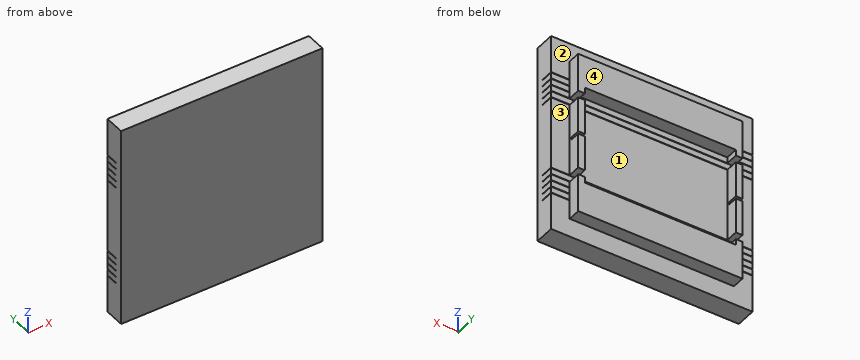
Autodesk Inventor part; units mm, degrees
ref_plane "YZ Plane" through (0, 0, 0) normal (1, 0, 0) x (0, 1, 0)
ref_plane "XZ Plane" through (0, 0, 0) normal (0, 1, 0) x (-1, 0, 0)
ref_plane "XY Plane" through (0, 0, 0) normal (0, 0, 1) x (1, 0, 0)
sketch "Boceto1" plane through (0, 0, 0) normal (0, 1, 0) x (-1, 0, 0)
  line L0 (0, 0) -> (80, 0)
  line L1 (80, 0) -> (80, -80)
  line L2 (80, -80) -> (0, -80)
  line L3 (0, -80) -> (0, 0)
  line L4 (10, -70) -> (70, -70)
  line L5 (70, -70) -> (70, -10)
  line L6 (70, -10) -> (10, -10)
  line L7 (10, -10) -> (10, -70)
  line L8 (0, -12.375) -> (80, -12.375)
  line L9 (0, -14.95) -> (80, -14.95)
  line L10 (0, -17.525) -> (80, -17.525)
  line L11 (80, -20.1) -> (0, -20.1)
  line L12 (0, -22.675) -> (80, -22.675)
  line L13 (0, -12.575) -> (80, -12.575)
  line L14 (0, -15.15) -> (80, -15.15)
  line L15 (0, -17.725) -> (80, -17.725)
  line L16 (80, -20.3) -> (0, -20.3)
  line L17 (0, -22.875) -> (80, -22.875)
  line L18 (0, -25.25) -> (80, -25.25)
  line L19 (0, -25.45) -> (80, -25.45)
  line L20 (10, -40) -> (80, -40)
  line L21 (0, -67.625) -> (80, -67.625)
  line L22 (0, -65.05) -> (80, -65.05)
  line L23 (0, -62.475) -> (80, -62.475)
  line L24 (80, -59.9) -> (0, -59.9)
  line L25 (0, -57.325) -> (80, -57.325)
  line L26 (0, -67.425) -> (80, -67.425)
  line L27 (0, -64.85) -> (80, -64.85)
  line L28 (0, -62.275) -> (80, -62.275)
  line L29 (80, -59.7) -> (0, -59.7)
  line L30 (0, -57.125) -> (80, -57.125)
  line L31 (0, -54.75) -> (80, -54.75)
  line L32 (0, -54.55) -> (80, -54.55)
  line L33 (72.625, -7.375) -> (7.375, -7.375)
  line L34 (7.375, -7.375) -> (7.375, -72.625)
  line L35 (7.375, -72.625) -> (72.625, -72.625)
  line L36 (72.625, -72.625) -> (72.625, -7.375)
  line L37 (7.375, 0) -> (0, 0)
  line L38 (7.375, -80) -> (0, -80)
  point P0 (10, -12.375)
  point P1 (70, -12.375)
  point P2 (10, -14.95)
  point P3 (70, -14.95)
  point P4 (10, -17.525)
  point P5 (70, -17.525)
  point P6 (70, -20.1)
  point P7 (10, -20.1)
  point P8 (10, -22.675)
  point P9 (70, -22.675)
  point P10 (10, -12.575)
  point P11 (70, -12.575)
  point P12 (10, -15.15)
  point P13 (70, -15.15)
  point P14 (10, -17.725)
  point P15 (70, -17.725)
  point P16 (70, -20.3)
  point P17 (10, -20.3)
  point P18 (10, -22.875)
  point P19 (70, -22.875)
  point P20 (10, -25.25)
  point P21 (70, -25.25)
  point P22 (10, -25.45)
  point P23 (70, -25.45)
  point P24 (10, -67.625)
  point P25 (70, -67.625)
  point P26 (10, -65.05)
  point P27 (70, -65.05)
  point P28 (10, -62.475)
  point P29 (70, -62.475)
  point P30 (70, -59.9)
  point P31 (10, -59.9)
  point P32 (10, -57.325)
  point P33 (70, -57.325)
  point P34 (10, -67.425)
  point P35 (70, -67.425)
  point P36 (10, -64.85)
  point P37 (70, -64.85)
  point P38 (10, -62.275)
  point P39 (70, -62.275)
  point P40 (70, -59.7)
  point P41 (10, -59.7)
  point P42 (10, -57.125)
  point P43 (70, -57.125)
  point P44 (10, -54.75)
  point P45 (70, -54.75)
  point P46 (10, -54.55)
  point P47 (70, -54.55)
  point P48 (72.625, -12.375)
  point P49 (7.375, -12.375)
  point P50 (72.625, -54.55)
  point P51 (72.625, -25.45)
  point P52 (70, -25.45)
  point P53 (70, -54.55)
  point P54 (7.375, -25.45)
  point P55 (7.375, -54.55)
  point P56 (10, -54.55)
  point P57 (10, -25.45)
  point P58 (10, -67.625)
  point P59 (7.375, -67.625)
  point P60 (72.625, -67.625)
  point P61 (70, -67.625)
  point P62 (7.375, -14.95)
  point P63 (72.625, -14.95)
  point P64 (72.625, -65.05)
  point P65 (70, -65.05)
  point P66 (10, -65.05)
  point P67 (7.375, -65.05)
  point P68 (70, -67.425)
  point P69 (10, -67.425)
  point P70 (10, -12.575)
  point P71 (70, -12.575)
  point P72 (72.625, -64.85)
  point P73 (7.375, -64.85)
  point P74 (7.375, -15.15)
  point P75 (70, -15.15)
  point P76 (7.375, -62.475)
  point P77 (10, -64.85)
  point P78 (10, -62.475)
  point P79 (72.625, -62.475)
  point P80 (70, -62.475)
  point P81 (70, -64.85)
  point P82 (7.375, -17.525)
  point P83 (10, -15.15)
  point P84 (72.625, -17.525)
  point P85 (72.625, -20.1)
  point P86 (7.375, -20.1)
  point P87 (72.625, -59.9)
  point P88 (70, -59.9)
  point P89 (70, -62.275)
  point P90 (10, -62.275)
  point P91 (10, -59.9)
  point P92 (7.375, -59.9)
  point P93 (10, -17.725)
  point P94 (70, -17.725)
  point P95 (72.625, -57.325)
  point P96 (70, -57.325)
  point P97 (70, -59.7)
  point P98 (10, -59.7)
  point P99 (10, -57.325)
  point P100 (7.375, -57.325)
  point P101 (7.375, -22.675)
  point P102 (10, -20.3)
  point P103 (70, -20.3)
  point P104 (72.625, -22.675)
  dimension "d5" = 10
  dimension "d0" = 80
  dimension "d1" = 80
  dimension "d2" = 60
  dimension "d3" = 60
  dimension "d4" = 10
  dimension "d6" = 2.375
  dimension "d7" = 0.2
  dimension "d8" = 2.375
  dimension "d9" = 0.2
  dimension "d10" = 0.2
  dimension "d11" = 0.2
  dimension "d12" = 0.2
  dimension "d13" = 2.375
  dimension "d14" = 2.375
  dimension "d15" = 2.375
  dimension "d16" = 2.375
  dimension "d17" = 0.2
  dimension "d35" = 5
extrude "Extrusión1" add sketch "Boceto1" along normal blind 5 contours L0 L1 L8 L36 L33 L34 L3 | L8 L34 L13 L3 | L13 L34 L9 L3 | L34 L33 L36 L8 L5 L6 L7 | L8 L7 L13 L34 | L1 L13 L36 L8 | L13 L7 L9 L34 | L8 L5 L13 L7 | L7 L6 L5 L8 | L1 L9 L36 L13 | L36 L13 L5 L8 | L14 L34 L10 L3 | L13 L5 L9 L7 | L36 L9 L5 L13 | L14 L7 L10 L34 | L1 L10 L36 L14 | L15 L34 L11 L3 | L14 L5 L10 L7 | L36 L10 L5 L14 | L15 L7 L11 L34 | L1 L11 L36 L15 | L16 L34 L12 L3 | L15 L5 L11 L7 | L36 L11 L5 L15 | L16 L7 L12 L34 | L1 L12 L36 L16 | L17 L34 L18 L3 | L16 L5 L12 L7 | L36 L12 L5 L16 | L17 L7 L18 L34 | L1 L18 L36 L17 | L19 L34 L32 L3 | L17 L5 L18 L7 | L36 L18 L5 L17 | L19 L7 L32 L34 | L1 L20 L36 L19 | L31 L34 L30 L3 | L19 L5 L20 L7 | L1 L32 L36 L20 | L36 L20 L5 L19 | L31 L7 L30 L34 | L7 L20 L5 L32 | L36 L32 L5 L20 | L25 L34 L29 L3 | L31 L5 L30 L7 | L1 L30 L36 L31 | L25 L7 L29 L34 | L31 L36 L30 L5 | L24 L34 L28 L3 | L25 L5 L29 L7 | L1 L29 L36 L25 | L24 L7 L28 L34 | L25 L36 L29 L5 | L23 L34 L27 L3 | L24 L5 L28 L7 | L1 L28 L36 L24 | L23 L7 L27 L34 | L24 L36 L28 L5 | L22 L34 L26 L3 | L23 L5 L27 L7 | L1 L27 L36 L23 | L26 L34 L21 L3 | L22 L7 L26 L34 | L23 L36 L27 L5 | L21 L34 L35 L36 L1 L2 L3 | L26 L7 L21 L34 | L22 L5 L26 L7 | L1 L26 L36 L22 | L21 L7 L4 L5 L36 L35 L34 | L26 L5 L21 L7 | L22 L36 L26 L5 | L1 L21 L36 L26 | L21 L5 L4 L7 | L26 L36 L21 L5
sketch "Boceto2" plane through (0, 0, 0) normal (0, -1, 0) x (1, 0, 0)
  line L0 (0, -80) -> (-80, -80)
  line L1 (-80, 0) -> (0, 0)
  line L2 (-80, -80) -> (-80, 0)
  line L3 (-80, 0) -> (0, 0)
  line L4 (-80, -65.05) -> (0, -65.05) construction
  line L5 (0, 0) -> (0, -80)
  line L6 (-80, -80) -> (0, -80)
extrude "Extrusión4" add sketch "Boceto2" along normal blind 3
extrude "Extrusión5" add sketch "Boceto1" along normal blind 10 contours L34 L33 L36 L8 L5 L6 L7 | L8 L7 L13 L34 | L13 L7 L9 L34 | L8 L5 L13 L7 | L7 L6 L5 L8 | L36 L13 L5 L8 | L9 L7 L14 L34 | L13 L5 L9 L7 | L36 L9 L5 L13 | L14 L7 L10 L34 | L9 L5 L14 L7 | L36 L14 L5 L9 | L10 L7 L15 L34 | L14 L5 L10 L7 | L36 L10 L5 L14 | L15 L7 L11 L34 | L10 L5 L15 L7 | L36 L15 L5 L10 | L11 L7 L16 L34 | L15 L5 L11 L7 | L36 L11 L5 L15 | L16 L7 L12 L34 | L11 L5 L16 L7 | L36 L16 L5 L11 | L36 L12 L5 L16 | L19 L7 L32 L34 | L36 L20 L5 L19 | L36 L32 L5 L20 | L25 L7 L29 L34 | L29 L7 L24 L34 | L24 L7 L28 L34 | L29 L5 L24 L7 | L25 L36 L29 L5 | L28 L7 L23 L34 | L24 L5 L28 L7 | L29 L36 L24 L5 | L23 L7 L27 L34 | L28 L5 L23 L7 | L24 L36 L28 L5 | L27 L7 L22 L34 | L23 L5 L27 L7 | L28 L36 L23 L5 | L22 L7 L26 L34 | L27 L5 L22 L7 | L23 L36 L27 L5 | L26 L7 L21 L34 | L22 L5 L26 L7 | L27 L36 L22 L5 | L21 L7 L4 L5 L36 L35 L34 | L26 L5 L21 L7 | L22 L36 L26 L5 | L21 L5 L4 L7 | L26 L36 L21 L5
sketch "Boceto3" plane through (0, 10, 0) normal (0, 1, 0) x (1, 0, 0)
  line L0 (-7.375, 25.45) -> (-7.375, 54.55)
  line L1 (-7.375, 40) -> (-86.5517, 40)
  line L2 (-5, 39.5) -> (-84.1767, 39.5)
  line L3 (-5, 40.5) -> (-84.1767, 40.5)
  line L4 (-10, 54.55) -> (-10, 25.45)
  line L5 (-5, 40.5) -> (-5, 39.5)
  line L6 (-84.1767, 40.5) -> (-84.1767, 39.5)
  point P0 (0, 0)
  point P1 (-10, 40)
  point P2 (-10, 39.5)
  point P3 (-10, 40.5)
  point P4 (-7.375, 39.5)
  point P5 (-7.375, 40.5)
  dimension "d31" = 0.5
  dimension "d32" = 0.5
extrude "Extrusión6" cut sketch "Boceto3" against normal blind 4 contours L2 L4 L1 L0 | L1 L4 L3 L0 | L2 L6 L1 L4 | L1 L6 L3 L4
equation "\"d8\" = d6"
equation "\"d9\" = d7"
equation "\"d10\" = d9"
equation "\"d11\" = d7"
equation "\"d12\" = d7"
equation "\"d13\" = d6"
equation "\"d14\" = d6"
equation "\"d15\" = d6"
equation "\"d16\" = d6"
equation "\"d17\" = d7"
properties part number "Cortador Ancho PDMS4"
Can you work these out from the model? Positions are in its coordinate system, mm. Face numbers are marked on the shaded views. A direction names the side the tool comes from. Give positions to 0.01 mm unless a question says otherwise; leave off trailing zeros. Order: outer loops, then holes, each group sorted by start corner. A loop starts at its lowest first (then second) coordinate and runs counter-clockwise, first axis right, second up. Notation, with made-up numbers: M 23,1 L 54,1 A21 cw 54,20 Z; hole C 30.5,16.5 d3. An arc over 180 degrees is marked long. Use one line per item in the form item = value.
Item 1: Will this pin go through, and if not, where does the flat tip stop? pin 1 Ø2.5 at (x, z) = (-2, -59) entering from +Y.
Values follow:
pin_1 = 5
Item 2: For the marked faces 3 and 4, which set-ups out of +Z, -Z, +X, -X, +Y, -Y let a thin tool reach every point of the face, with its end or its side?
Values follow:
face_3 = +Z, -Z, +X, +Y
face_4 = +Z, -Z, +X, -X, +Y
Item 3: If I drill on line 1 along Z through (x, y) = (-69.5, 2.25) (3 decimals); line 2 along Z through (x, y) = (-39.5, 8.75) (3 decimals); line 3 along Y through (x, z) = (-61, -7), over which ranges is the centre line in solid material (lowest first)? Write a range as [from, to].
Values follow:
line_1 = [-80, -57.325], [-57.125, -54.75], [-54.55, -25.45], [-25.25, -22.875], [-22.675, 0]
line_2 = [-72.625, -59.7], [-20.3, -7.375]
line_3 = [-3, 5]
Item 4: If we section it at C-C, the plane x = -22: Write out the boundary of the cut face in (y, z) (3 decimals).
Values follow:
outline = M -3,-80 L 5,-80 L 5,-72.625 L 10,-72.625 L 10,-59.7 L 5,-59.7 L 5,-57.325 L 0,-57.325 L 0,-57.125 L 5,-57.125 L 5,-54.75 L 0,-54.75 L 0,-54.55 L 5,-54.55 L 5,-25.45 L 0,-25.45 L 0,-25.25 L 5,-25.25 L 5,-22.875 L 0,-22.875 L 0,-22.675 L 5,-22.675 L 5,-20.3 L 10,-20.3 L 10,-7.375 L 5,-7.375 L 5,0 L -3,0 Z
Item 5: Thinking about a two-plate mould opening in X: for the marked faces 1 and 2, which applies, pulls with the +X half, pulls with the -X half, needs draft (parallel to the pull), parting line crosses it, or undercut?
Values follow:
face_1 = undercut
face_2 = needs draft
Item 6: If we section it at A-A, the plane y = 8.75: Count the separate pieces of the cut face and the enclosed holes in it, and give its area (3 significant figures).
Values follow:
separate_pieces = 6
enclosed_holes = 0
area = 1,860 mm^2
Item 7: If we section it at B-B, the plane z = -27.5: Write out the boundary of the cut face in (x, y) (3 decimals).
Values follow:
outline = M -80,-3 L 0,-3 L 0,5 L -7.375,5 L -7.375,10 L -10,10 L -10,5 L -70,5 L -70,10 L -72.625,10 L -72.625,5 L -80,5 Z
